Print and shaded views of the part. All mm, measured from the part's lowest x, y and z. A direction names the side the tool comes from. Give positions to 0.01 mm unless a question says otherwise; leave off trailing zeros. Loops run counter-clockwise (first coordinate to the right, second up) from the corner with the lowest first, then second, coordinate; pieces in that order, holes last.
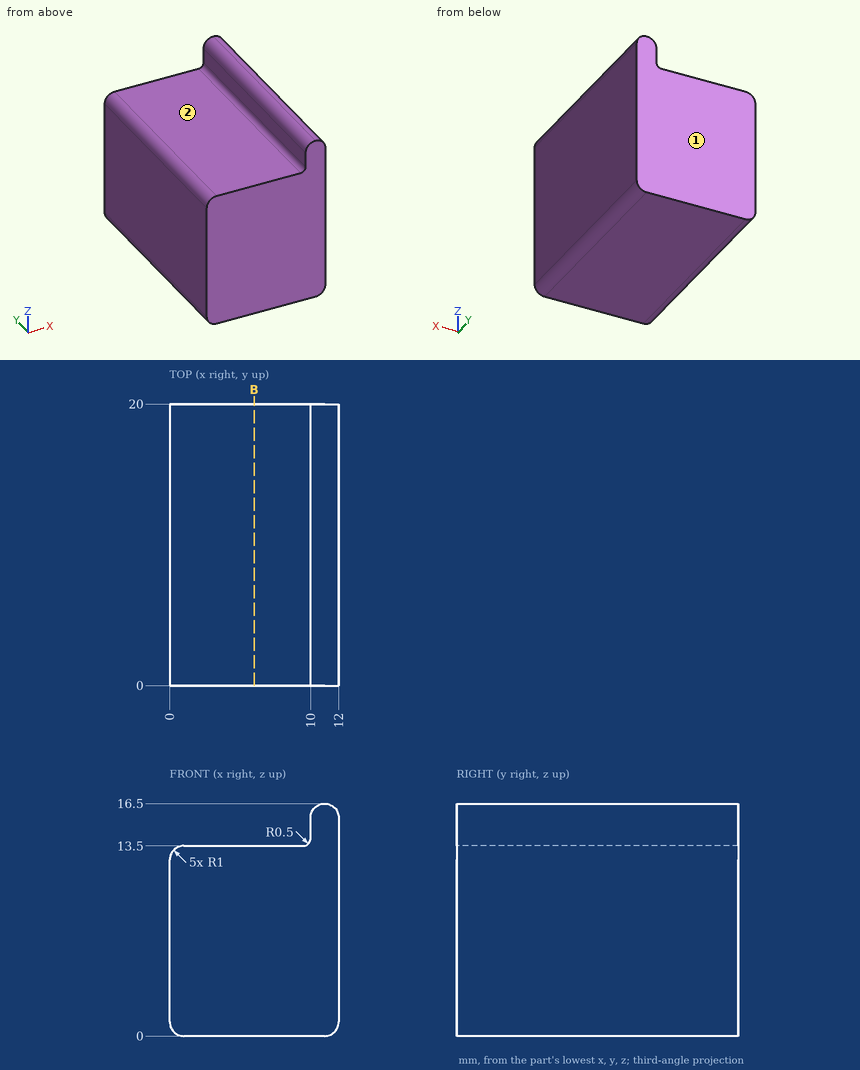
1. Probe line 1 along Z through (x, y) = (5, 1.75); line 2 along X through (y, z) = (7.5, 14.75); line 3 along Z through (x, y) = (10.75, 1.75). List the from-to ranges inside material, lowest first.
Responses:
line 1: z = 0 to 13.5
line 2: x = 10 to 12
line 3: z = 0 to 16.47
2. Saw through at B-B, the plane x = 6. List the corners of the cut face in (y, z).
Responses:
outline: (0, 0) - (20, 0) - (20, 13.5) - (0, 13.5) - close
3. Drop flat-ended pins along their axis: pin 1 (1.7 mm diameter, centred on y = 5.5, z = 15, fed in from -X); pin 2 (6 mm diameter, centred on x = 6, y = 13, fed in from +Z). Give the stop position or say it passes through.
Responses:
pin 1: stops at x = 10
pin 2: stops at z = 13.5
4. Tool access for the marked faces 1 and 2: list every direction of +Z, -Z, +X, -X, +Y, -Y with a clear straight run to the whole face (end or side of a thin tool).
Responses:
face 1: +Z, -Z, +X, -X, +Y
face 2: +Z, -X, +Y, -Y
